Can you work these out from the model? Positions are in its coordinate system, mm. Face numbers are marked on the shaded views. A direction names the side the tool comes from. Coordinates: 2 decimals unless noted, no trailing zeros. Order: outer loops, then holes, each group sorted by start corner. A loop starts at its lowest first (then second) coordinate and runs counter-clockwise, first axis right, second up. Notation, with made-up numbers: (59, 11.5) -> (72, 11.5) arc R11 ccw to (72, 18.5) -> close; hole circle Ø4 at (50.25, -11.75). An arc over 180 degrees is marked (long way). Answer as CSV lines item,"result".
from build123d import *

# Parameters (mm, degrees)
ESQUISSE1_R        = 4
BOSS_EXTRU_1_DEPTH = 1.25
ESQUISSE2_R        = 4.5
BOSS_EXTRU_2_DEPTH = 1.8
BOSS_EXTRU_3_START = 0.7
ESQUISSE3_R        = 4.5
BOSS_EXTRU_3_DEPTH = 0.7


with BuildPart() as part:
    # Esquisse1 → Boss.-Extru.1 (new, symmetric)
    with BuildSketch(Plane(origin=(0, 0, 0), x_dir=(1, 0, 0), z_dir=(0, 1, 0))):
        with Locations(Location((0, 0, 0), (0, 0, 270))):
            Circle(ESQUISSE1_R)
    extrude(amount=BOSS_EXTRU_1_DEPTH, both=True)

    # Esquisse2 → Boss.-Extru.2 (add)
    with BuildSketch(Plane(origin=(0, 1.25, 0), x_dir=(1, 0, 0), z_dir=(0, 1, 0))):
        with Locations(Location((0, 0, 0), (0, 0, 270))):
            Circle(ESQUISSE2_R)
    extrude(amount=BOSS_EXTRU_2_DEPTH)

    # Esquisse3 → Boss.-Extru.3 (add)
    with BuildSketch(Plane(origin=(0, -1.25, 0), x_dir=(-1, 0, 0), z_dir=(0, -1, 0)).offset(BOSS_EXTRU_3_START)):
        with Locations(Location((0, 0, 0), (0, 0, 270))):
            Circle(ESQUISSE3_R)
    extrude(amount=-BOSS_EXTRU_3_DEPTH)

    # Esquisse4 → Perçage1 (revolve, cut)
    with BuildSketch(Plane(origin=(0, -1.95, 0), x_dir=(0, 0, -1), z_dir=(1, 0, 0))):
        Polygon((0, 0), (0, 10.600860619), (1, 10), (1, 1.600860619), (2, 1), (2, 0), align=None)
    revolve(axis=Axis((0, -8.080023899, 0), (0, 1, 0)), mode=Mode.SUBTRACT)


solid = part.part
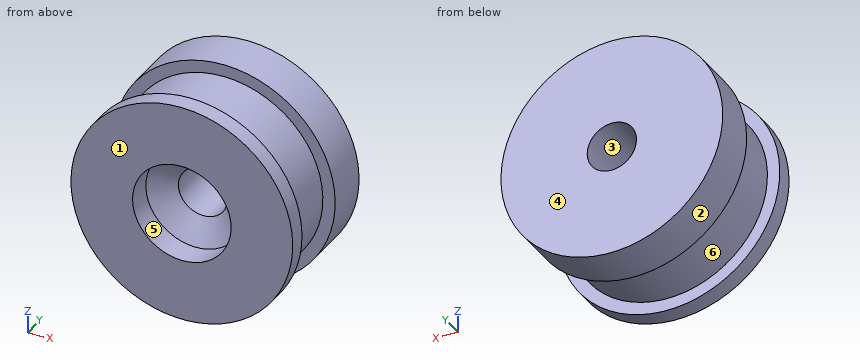
Q1. Imagine slicing it at D-D (x = 3.75). List the corners of the cut face in (y, z) for me.
Solution:
outline,"(-1.95, -2.49) -> (-1.25, -2.49) -> (-1.25, -1.39) -> (1.25, -1.39) -> (1.25, -2.49) -> (3.05, -2.49) -> (3.05, 2.49) -> (1.25, 2.49) -> (1.25, 1.39) -> (-1.25, 1.39) -> (-1.25, 2.49) -> (-1.95, 2.49) -> close"
Q2. Imagine slicing it at B-B (x = 0). List the corners of the cut face in (y, z) for me.
Solution:
outline,"(-1.95, -4.5) -> (-1.25, -4.5) -> (-1.25, -4) -> (1.25, -4) -> (1.25, -4.5) -> (3.05, -4.5) -> (3.05, -1) -> (-0.35, -1) -> (-0.95, -2) -> (-1.95, -2) -> close; (-1.95, 2) -> (-0.95, 2) -> (-0.35, 1) -> (3.05, 1) -> (3.05, 4.5) -> (1.25, 4.5) -> (1.25, 4) -> (-1.25, 4) -> (-1.25, 4.5) -> (-1.95, 4.5) -> close"
Q3. We'd pull the mould along Z, two halves only. Please class the marked faces 1, 2 and 3: pulls with the +Z half, pulls with the -Z half, needs draft (parallel to the pull), parting line crosses it, or undercut.
Solution:
face 1,"needs draft"
face 2,"parting line crosses it"
face 3,"undercut"
Q4. Imagine slicing it at C-C (y = -1.6). List the corners of the cut face in (x, z) for me, and give its area (3 significant figures).
Solution:
outline,"circle Ø9 at (0, 0); hole circle Ø4 at (0, 0)"
area,"51.1 mm2"
Q5. Which directions (+Z, -Z, +X, -X, +Y, -Y) give clear straight access to the entire face, cutting with the end or side of a thin tool? Please do the marked faces 4, 5 and 6.
Solution:
face 4,"+Z, -Z, +X, -X, +Y"
face 5,"-Y"
face 6,"none"
Q6. If I drill on line 1 (X direction, y = 1.45, z = 0); line 2 (Y direction, x = 0.25, z = 4.25); line 3 (X direction, y = -1.6, z = 0), over which ranges is the centre line in solid material (lowest first)?
Solution:
line 1,"-4.5 to -1, 1 to 4.5"
line 2,"-1.95 to -1.25, 1.25 to 3.05"
line 3,"-4.5 to -2, 2 to 4.5"
Q7. Imagine slicing it at A-A (z = 0). List the corners of the cut face in (x, y) for me, and give its area (3 significant figures).
Solution:
outline,"(-4.5, -1.95) -> (-2, -1.95) -> (-2, -0.95) -> (-1, -0.35) -> (-1, 3.05) -> (-4.5, 3.05) -> (-4.5, 1.25) -> (-4, 1.25) -> (-4, -1.25) -> (-4.5, -1.25) -> close; (1, -0.35) -> (2, -0.95) -> (2, -1.95) -> (4.5, -1.95) -> (4.5, -1.25) -> (4, -1.25) -> (4, 1.25) -> (4.5, 1.25) -> (4.5, 3.05) -> (1, 3.05) -> close"
area,"29.9 mm2"
Q8. For P1, Ø1.5, axis at y = 1.5, z = 2, coming from the -X side; P2, Ø1.5, axis at x = 1, y = 0, coming from the -Z side; P3, Ø1.6, axis at x = 0, z = 0, coming from the +Y side; P4, Ø2.5, axis at x = 0, z = 0, coming from the -Y side, each with a flat end and sliding along its axis, tell me the tip position at first contact or that it passes through.
Solution:
P1,"x = -4.32"
P2,"z = -3.99"
P3,"through"
P4,"y = -0.5"
